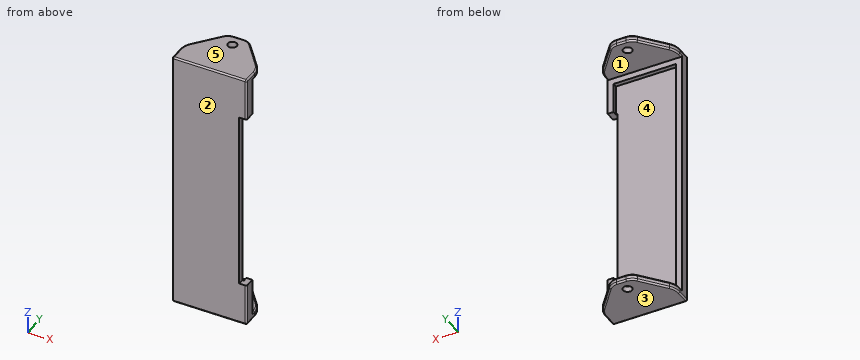
```python
from build123d import *

# Parameters (mm, degrees)
SKETCH_1_W          = 25
SKETCH_1_H          = 3.5
EXTRUDE_1_DEPTH     = 84.3
SHELL_1_T           = -2
SKETCH_2_W          = 2.5
SKETCH_2_H          = 60
CUT_EXTRUDE_1_DEPTH = 88.998522715
EXTRUDE_2_DEPTH     = 2
EXTRUDE_3_DEPTH     = 2
SKETCH_5_R          = 1.5
CUT_EXTRUDE_2_DEPTH = 94.519463215
FILLET_1_R          = 4
FILLET_2_R          = 6
FILLET_3_R          = 0.5
FILLET_4_R          = 0.5


with BuildPart() as part:
    # 草图1 → 凸台-拉伸1 (new body)
    with BuildSketch(Plane.XY):
        with Locations((12.5, 1.75)):
            Rectangle(SKETCH_1_W, SKETCH_1_H)
    extrude(amount=EXTRUDE_1_DEPTH)

    # 抽壳1
    shell_1_openings = [part.faces().sort_by_distance(p)[0] for p in [
        (12.5, 3.5, 42.15),
    ]]
    offset(amount=SHELL_1_T, openings=shell_1_openings, kind=Kind.INTERSECTION)

    # 草图2 → 切除-拉伸1 (cut, through all)
    with BuildSketch(Plane.XZ):
        with Locations((23.75, 42.15)):
            Rectangle(SKETCH_2_W, SKETCH_2_H)
    extrude(amount=-CUT_EXTRUDE_1_DEPTH, mode=Mode.SUBTRACT)

    # 草图3 → 凸台-拉伸2 (add)
    with BuildSketch(Plane(origin=(0, 0, 0), x_dir=(-1, 0, 0), z_dir=(0, 0, -1))):
        Polygon((-25, 7), (-16, 18), (-9, 18), (0, 7), (0, 0), (-25, 0), align=None)
    extrude(amount=EXTRUDE_2_DEPTH)

    # 草图4 → 凸台-拉伸3 (add)
    with BuildSketch(Plane.XY.offset(84.3)):
        Polygon((0, 0), (0, 7), (9, 18), (16, 18), (25, 7), (25, 0), align=None)
    extrude(amount=EXTRUDE_3_DEPTH)

    # 草图5 → 切除-拉伸2 (cut, through all)
    with BuildSketch(Plane.XY.offset(86.3)):
        with Locations((12.5, 14)):
            Circle(SKETCH_5_R)
    extrude(amount=-CUT_EXTRUDE_2_DEPTH, mode=Mode.SUBTRACT)

    # 圆角1
    fillet_1_edges = [part.edges().sort_by_distance(p)[0] for p in [
        (9, 18, -1),
        (16, 18, -1),
        (16, 18, 85.3),
        (9, 18, 85.3),
    ]]
    fillet(fillet_1_edges, radius=FILLET_1_R)

    # 圆角2
    fillet_2_edges = [part.edges().sort_by_distance(p)[0] for p in [
        (25, 7, -1),
        (0, 7, -1),
        (25, 7, 85.3),
        (0, 7, 85.3),
    ]]
    fillet(fillet_2_edges, radius=FILLET_2_R)

    # 圆角3
    fillet_3_edges = [part.edges().sort_by_distance(p)[0] for p in [
        (4.577971759, 12.595298817, 86.3),
        (9.182595707, 17.61467873, 86.3),
        (15.817404293, 17.61467873, 86.3),
        (0, 2.429109865, 86.3),
        (0, 4.179109865, 84.3),
        (20.422028241, 12.595298817, 84.3),
        (24.650772636, 6.87533862, 84.3),
        (0.349227364, 6.87533862, 84.3),
        (20.422028241, 12.595298817, 86.3),
        (24.650772636, 6.87533862, 86.3),
        (0.349227364, 6.87533862, 86.3),
        (25, 2.429109865, -2),
        (25, 4.179109865, 0),
        (4.577971759, 12.595298817, 0),
        (0.349227364, 6.87533862, 0),
        (24.650772636, 6.87533862, 0),
        (4.577971759, 12.595298817, -2),
        (0.349227364, 6.87533862, -2),
        (24.650772636, 6.87533862, -2),
        (0, 4.179109865, 0),
        (0, 2.429109865, -2),
        (25, 4.179109865, 84.3),
        (25, 2.429109865, 86.3),
        (20.422028241, 12.595298817, 0),
        (20.422028241, 12.595298817, -2),
        (12.5, 18, 0),
        (9.182595707, 17.61467873, 0),
        (15.817404293, 17.61467873, 0),
        (12.5, 18, -2),
        (9.182595707, 17.61467873, -2),
        (15.817404293, 17.61467873, -2),
        (12.5, 18, 84.3),
        (12.5, 18, 86.3),
        (4.577971759, 12.595298817, 84.3),
        (9.182595707, 17.61467873, 84.3),
        (15.817404293, 17.61467873, 84.3),
    ]]
    fillet(fillet_3_edges, radius=FILLET_3_R)

    # 圆角4
    fillet_4_edges = [part.edges().sort_by_distance(p)[0] for p in [
        (25, 0, 78.975),
        (24.853553391, 0, -1.853553391),
        (12.5, 0, -2),
        (0.146446609, 0, -1.853553391),
        (0, 0, 42.15),
        (0.146446609, 0, 86.153553391),
        (24.853553391, 0, 86.153553391),
        (12.5, 0, 86.3),
    ]]
    fillet(fillet_4_edges, radius=FILLET_4_R)


solid = part.part
```
Input: part model. Units: mm. Frame: model coordinates. Face numbers are marked on the shaded views. A direction names the side the tool comes from. Coordinates: 2 decimals unless noted, no trailing zeros. Loops run counter-clockwise (first coordinate to the right, second up) from the corner with the lowest first, then second, coordinate; pieces in that order, holes last. Notation, with made-up numbers: M 18.25,38 L 60.25,38 A28 cw 60.25,57 Z; hole C 50,25 d2. An arc over 180 degrees is marked long. Use a Markdown table: item, result. Add a question column.
1) Draft query along Z for the marked faces 3, 4 and 5. Return one class per face: +Z half, -Z half, draft (parallel to the pull), parting line (faces both ways), or undercut.
2) Pin query (flat end, axial travel): P1, Ø6, axis at x = 3, z = 73.5, coming from the +Y side; P2, Ø12.5, axis at x = 13, z = 22, coming from the +Y side; P3, Ø1, axis at y = 1.5, z = 31.5, coming from the +X side; P4, Ø10, axis at y = 5, z = 61, coming from the -X side. Return the tip coordinate at first contact, or that it passes through.
3) Section C-C, the plane y = 14. Give the number of separate pieces and of enclosed holes in the cut face, plus the area to 3 significant figures.
4) Section B-B, the plane z = 17. Return the cut outline in (x, y), plus the area to 3 significant figures.
5) Section A-A, the plane x = 12.5. Return the cut outline in (y, z), plus the area to 3 significant figures.
6) Line query: L1, parallel to Y at x = 12.5, z = 85.8; L2, parallel to Z at x = 13.5, y = 8.5; L3, parallel to Y at x = 20, z = 70.5. Output: solid intervals per line, ascending. Write a range as from..to.
7) Set-up query: the marked faces 1 and 2. Return all of +Z, -Z, +X, -X, +Y, -Y with unobstructed straight access to the full face (end or side cutting, diameter ignored); none if empty.
Answer below:
| question | item | result |
|---|---|---|
| 1 | face 3 | -Z half |
| 1 | face 4 | undercut |
| 1 | face 5 | +Z half |
| 2 | P1 | y = 3.5 |
| 2 | P2 | y = 2 |
| 2 | P3 | x = 22.5 |
| 2 | P4 | x = 0 |
| 3 | separate pieces | 4 |
| 3 | enclosed holes | 0 |
| 3 | area | 41.6 mm2 |
| 4 | outline | M 0,0.5 A0.5 ccw 0.5,0 L 22.5,0 L 22.5,2 L 2,2 L 2,3.5 L 0,3.5 Z |
| 4 | area | 47.9 mm2 |
| 5 | outline | M 0,-1.5 A0.5 ccw 0.5,-2 L 12.5,-2 L 12.5,0 L 3.5,0 L 3.5,2 L 2,2 L 2,82.3 L 3.5,82.3 L 3.5,84.3 L 12.5,84.3 L 12.5,86.3 L 0.5,86.3 A0.5 ccw 0,85.8 Z; M 15.5,-2 L 17.5,-2 A0.5 ccw 18,-1.5 L 18,-0.5 A0.5 ccw 17.5,0 L 15.5,0 Z; M 15.5,84.3 L 17.5,84.3 A0.5 ccw 18,84.8 L 18,85.8 A0.5 ccw 17.5,86.3 L 15.5,86.3 Z |
| 5 | area | 234 mm2 |
| 6 | L1 | 0..12.5, 15.5..18 |
| 6 | L2 | -2..0, 84.3..86.3 |
| 6 | L3 | 0..2 |
| 7 | face 1 | +X, -X, +Y |
| 7 | face 2 | +Z, -Z, +X, -X, -Y |
